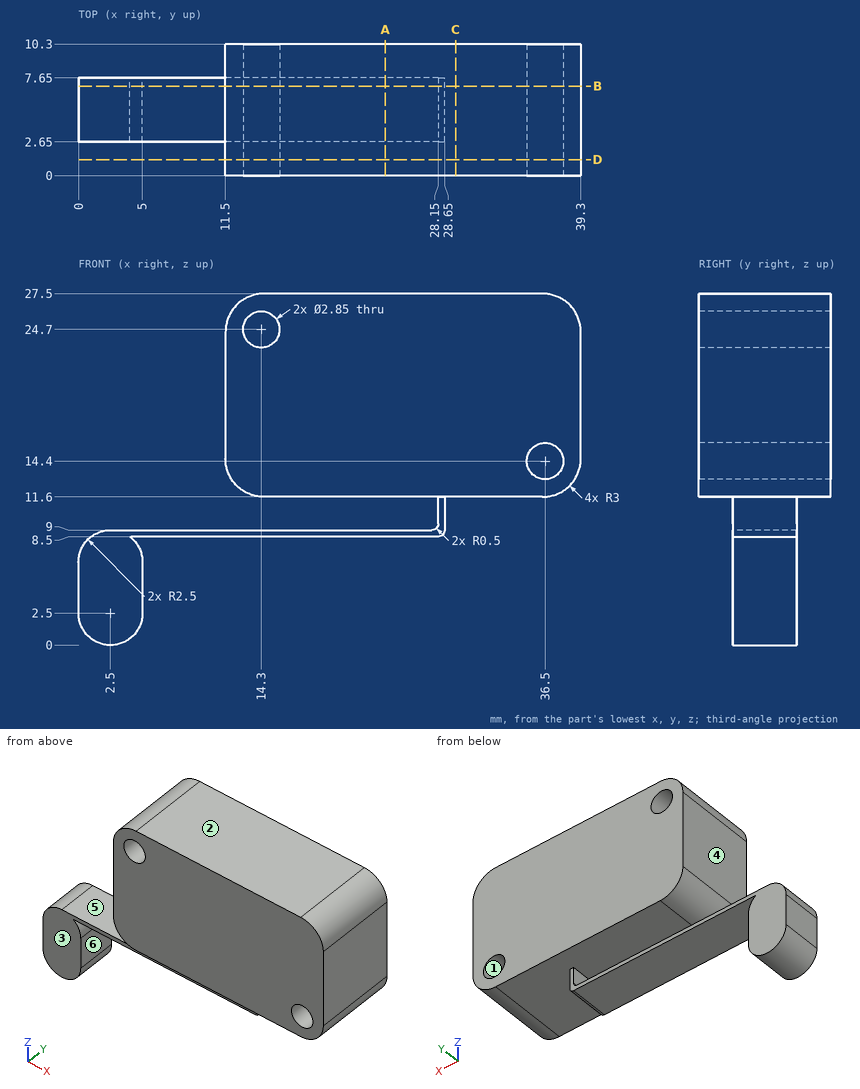
Can you work these out from the drawing? Everything is in mm from the part's minimum corner. A direction names the side the tool comes from. Coordinates: 2 decimals unless noted, no trailing zeros. Loops run counter-clockwise (first coordinate to the right, second up) from the corner with the lowest first, then second, coordinate; pieces in that order, holes last. Notation, with made-up numbers: M -5,17 L 20,17 A20 ccw 20,56 Z; hole C 3.25,-14.5 d8. An arc over 180 degrees is marked long. Put each result on its own line as item: value. Start each with the question number.
(1) I need wall thicknesses on line 1 (Z direction, x = 14.3, y = 4.75) (3 decimals); line 2 (X direction, y = 5, z = 14.4) (3 decimals); line 3 (Z direction, x = 14.3, y = 7.75) (3 decimals). Which ranges of each line are inside material? Lowest first, please. Write a range as from..to.
(2) Suppose I cut it at C-C on x = 29.5. Please give me the cut outline in (y, z).
(3) Suppose I cut it at B-B on y = 7. Please give me the cut outline in (x, z) (3 decimals).
(4) Will these pins go through, and if not, where does the flat tip stop? P1, Ø3.5, axis at x = 14.3, z = 24.7, coming from the +Y side; P2, Ø1.2, axis at y = 4, z = 4.5, coming from the +X side; P3, Ø1, axis at y = 1.5, z = 13, coming from the -X side; P4, Ø1, axis at x = 9, y = 7, coming from the +Z side.
(5) For the marked faces 4, 5 and 6, which set-ups out of +Z, -Z, +X, -X, +Y, -Y let a thin tool reach every point of the face, with its end or its side?
(6) Suppose I cut it at A-A on x = 24. Please give me the cut outline in (y, z).
(7) Thinking about a two-plate mould opening in Z: for the marked faces 1, 2 and 3, which applies, pulls with the +Z half, pulls with the -Z half, needs draft (parallel to the pull), parting line crosses it, or undercut?
(8) Suppose I cut it at D-D on y = 1.25. Please give me the cut outline in (x, z) (3 decimals).
Solutions:
1. line 1: z = 8.5..9, 11.607..23.275, 26.125..27.493
1. line 2: x = 11.507..35.075, 37.925..39.293
1. line 3: z = 11.607..23.275, 26.125..27.493
2. outline: M 0,11.6 L 10.3,11.6 L 10.3,27.5 L 0,27.5 Z
3. outline: M 0,2.5 A2.5 ccw 5,2.5 L 5,6.5 A2.5 ccw 4,8.5 L 28.15,8.5 A0.5 ccw 28.65,9 L 28.65,11.6 L 36.3,11.6 A3 ccw 39.3,14.6 L 39.3,24.5 A3 ccw 36.3,27.5 L 14.5,27.5 A3 ccw 11.5,24.5 L 11.5,14.6 A3 ccw 14.5,11.6 L 28.15,11.6 L 28.15,9.5 A0.5 cw 27.65,9 L 2.5,9 A2.5 ccw 0,6.5 Z; hole C 14.3,24.7 d2.85; hole C 36.5,14.4 d2.85
4. P1: stops at y = 10.3
4. P2: stops at x = 5
4. P3: stops at x = 11.71
4. P4: stops at z = 9
5. face 4: +Z, -X, +Y, -Y
5. face 5: -X, +Y, -Y
5. face 6: -Z, +X, +Y, -Y
6. outline: M 0,11.6 L 10.3,11.6 L 10.3,27.5 L 0,27.5 Z; M 2.65,8.5 L 7.65,8.5 L 7.65,9 L 2.65,9 Z
7. face 1: undercut
7. face 2: pulls with the +Z half
7. face 3: needs draft
8. outline: M 11.5,14.6 A3 ccw 14.5,11.6 L 36.3,11.6 A3 ccw 39.3,14.6 L 39.3,24.5 A3 ccw 36.3,27.5 L 14.5,27.5 A3 ccw 11.5,24.5 Z; hole C 14.3,24.7 d2.85; hole C 36.5,14.4 d2.85
